Work out the finished part from the listing and answer in its coordinate system (mm). A direction names the side the tool comes from. Give positions to 0.01 mm unless a question says otherwise; leave off trailing zeros. Write each loop counter-clockwise with the first axis right and the second up, starting at its lowest first coordinate (ties: lowest second). Pieces come first, ordered by that corner, then holes.
1) Find section D-D (y = 7). Determine the outline of the cut face in (x, z), plus the area to 3 significant figures.
2) Straight lines are drawn through the part: probe 1 along X at (y, z) = (1.55, -6.35); probe 2 along Y at (x, z) = (26, -7.75). For each, find the intervals that lie inside material, in ascending order.
3) Find section B-B (z = -7). Determine the outline of the cut face in (x, y).
4) Find section A-A (y = 31.75). Determine the outline of the cut face in (x, z).
5) Determine the mould class of faces 1 (the face through (3, 10, 0)), 2 (the face through (19, 0, -6)), 3 (the face through (1.878, 14.456, -5.23)), 4 (the face through (33.783, 1.878, -5.898)) for opening direction Z: pulls with the +Z half, pulls with the -Z half, needs draft (parallel to the pull), parting line crosses it, or undercut.
6) Find section C-C (z = -11.25). Determine the outline of the cut face in (x, y).
7) Given pin 1 Ø2 at (x, z) = (30, -11) entering from -Y; pin 2 Ø6.5 at (x, z) = (31.75, -6.35) entering from +Y; pin 3 Ø6.5 at (y, z) = (23, -9) entering from +X, each flat-ended and moving along its own axis, determine where each tip first touches the part or whether it passes through.
8) A tool of negligible diameter and unlimited length cuts with its end or side. For faces 5 (the face through (3.81, 21, -6)), 6 (the face through (1.88, 29.9, -5.39)), from which of +Z, -Z, +X, -X, +Y, -Y can it reach the whole face along a straight path? Write none if from no direction.
```python
from build123d import *

# Parameters (mm, degrees)
SKETCH1_W           = 38.1
SKETCH1_H           = 12.7
SKETCH1_R           = 2.0828
BOSS_EXTRUDE1_DEPTH = 3.81
SKETCH2_W           = 12.7
SKETCH2_H           = 38.1
SKETCH2_R           = 2.0828
BOSS_EXTRUDE2_DEPTH = 3.81


with BuildPart() as part:
    # Sketch1 → Boss-Extrude1 (new body)
    with BuildSketch(Plane(origin=(0, 0, 0), x_dir=(1, 0, 0), z_dir=(0, 1, 0))):
        with Locations((19.05, 6.35)):
            Rectangle(SKETCH1_W, SKETCH1_H)
        with Locations(Location((12.7, 6.35, 0), (0, 0, 90))):
            Circle(SKETCH1_R, mode=Mode.SUBTRACT)
        with Locations(Location((31.75, 6.35, 0), (0, 0, 90))):
            Circle(SKETCH1_R, mode=Mode.SUBTRACT)
    extrude(amount=BOSS_EXTRUDE1_DEPTH)

    # Sketch2 → Boss-Extrude2 (add)
    with BuildSketch(Plane.ZY):
        with Locations((-6.35, 19.05)):
            Rectangle(SKETCH2_W, SKETCH2_H)
        with Locations((-6.35, 31.75)):
            Circle(SKETCH2_R, mode=Mode.SUBTRACT)
        with Locations((-6.35, 12.7)):
            Circle(SKETCH2_R, mode=Mode.SUBTRACT)
    extrude(amount=-BOSS_EXTRUDE2_DEPTH)


solid = part.part
```
Results:
1. outline: (0, -12.7) - (3.81, -12.7) - (3.81, 0) - (0, 0) - close
1. area: 48.4 mm2
2. probe 1: x = 0 to 10.62, 14.78 to 29.67, 33.83 to 38.1
2. probe 2: y = 0 to 3.81
3. outline: (0, 0) - (10.72, 0) - (10.72, 3.81) - (3.81, 3.81) - (3.81, 10.72) - (0, 10.72) - close; (0, 14.68) - (3.81, 14.68) - (3.81, 29.77) - (0, 29.77) - close; (0, 33.73) - (3.81, 33.73) - (3.81, 38.1) - (0, 38.1) - close; (14.68, 0) - (29.77, 0) - (29.77, 3.81) - (14.68, 3.81) - close; (33.73, 0) - (38.1, 0) - (38.1, 3.81) - (33.73, 3.81) - close
4. outline: (0, -12.7) - (3.81, -12.7) - (3.81, -8.43) - (0, -8.43) - close; (0, -4.27) - (3.81, -4.27) - (3.81, 0) - (0, 0) - close
5. face 1: pulls with the +Z half
5. face 2: needs draft
5. face 3: undercut
5. face 4: undercut
6. outline: (0, 0) - (38.1, 0) - (38.1, 3.81) - (3.81, 3.81) - (3.81, 38.1) - (0, 38.1) - close
7. pin 1: stops at y = 0
7. pin 2: stops at y = 3.81
7. pin 3: stops at x = 3.81
8. face 5: +Z, -Z, +X, +Y
8. face 6: +X, -X
